```python
from build123d import *

# Parameters (mm, degrees)
F2_DEPTH = 12.7
F3_D     = 9.525


with BuildPart() as f2:
    # F1 (on Top) → F2 (new body)
    with BuildSketch(Plane.XY):
        with BuildLine():
            ThreePointArc((-122.0150568144, -68.2625), (-138.5539190608, -65.4948436404), (-153.2906597609, -57.4934462832))
            Line((-153.2906597609, -57.4934462832), (-236.4102435549, 7.4466898162))
            ThreePointArc((-236.4102435549, 7.4466898162), (-234.1628787728, 4.6714254371), (-233.3595565153, 1.1918544595))
            ThreePointArc((-233.3595565153, 1.1918544595), (-237.8174855377, -5.942323283), (-246.1838694757, -5.0629808973))
            Line((-246.1838694757, -5.0629808973), (-163.0642856817, -70.0031169967))
            ThreePointArc((-163.0642856817, -70.0031169967), (-143.7223135128, -80.5049510281), (-122.0150568144, -84.1375))
            Line((-122.0150568144, -84.1375), (-33.3375, -84.1375))
            ThreePointArc((-33.3375, -84.1375), (-4.1516676065, -72.0483323935), (7.9375, -42.8625))
            Line((7.9375, -42.8625), (7.9375, 0))
            ThreePointArc((7.9375, 0), (0, -7.9375), (-7.9375, 0))
            Line((-7.9375, 0), (-7.9375, -42.8625))
            ThreePointArc((-7.9375, -42.8625), (-15.3769877579, -60.8230122421), (-33.3375, -68.2625))
            Line((-33.3375, -68.2625), (-122.0150568144, -68.2625))
        make_face()
        with BuildLine():
            ThreePointArc((-233.3595565153, 1.1918544595), (-234.1628787728, 4.6714254371), (-236.4102435549, 7.4466898162))
            ThreePointArc((-236.4102435549, 7.4466898162), (-247.5518918721, 6.0786674199), (-246.1838694757, -5.0629808973))
            ThreePointArc((-246.1838694757, -5.0629808973), (-237.8174855377, -5.942323283), (-233.3595565153, 1.1918544595))
        make_face()
        with BuildLine():
            ThreePointArc((7.9375, 0), (0, 7.9375), (-7.9375, 0))
            ThreePointArc((-7.9375, 0), (0, -7.9375), (7.9375, 0))
        make_face()
    extrude(amount=F2_DEPTH)

    # F3 (through all)
    with Locations(Plane(origin=(0, 0, 0), x_dir=(1, 0, 0), z_dir=(0, 0, -1))):
        with Locations((-241.2970565153, -1.1918544595), (0, 0)):
            Hole(F3_D / 2)


solid = f2.part
```
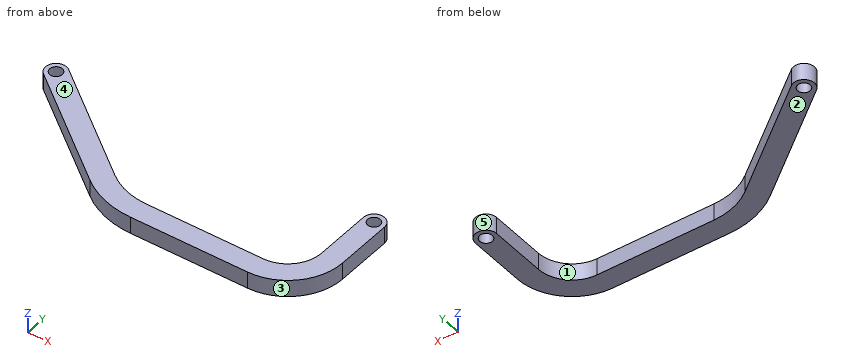
CAD build for the part. Positions are in the model's coordinates, mm. Face numbers are marked on the shaded views. A direction names the side the tool comes from. Round coordinates to 2 decimals unless told otherwise and drop trailing zeros. Order: outer loops, then holes, each group sorted by start corner. A loop starts at its lowest first (then second) coordinate and runs counter-clockwise, first axis right, second up.
Item 1: Saw through at D-D on x = -54. Write the cut outline in (y, z), then the cut area to 3 significant figures.
Item 2: Probe line 1 along Y through (x, z) = (-34.5, 6.25); line 2 along X through (y, z) = (-12.5, 1.5); line 3 along X through (y, z) = (-47.5, 1). List the from-to ranges inside material, lowest first.
Item 3: Saw through at A-A on x = 0. Write the cut outline in (y, z).
Item 4: Pin check, flat tip, straight feed: pin 1 (4 mm diameter, centred on x = -95.5, z = 5.5, fed in from +Y). Stop position of the tip, or through.
Item 5: Saw through at C-C on y = -17.5. Write the cut outline in (x, z), then the cut area to 3 significant figures.
Item 6: Saw through at B-B on z = 6. State how many separate pieces and enclosed holes the cut face has, then the cut area to 3 significant figures.
Item 7: Tool access for the marked faces 1 and 2: list every direction of +Z, -Z, +X, -X, +Y, -Y with a clear straight run to the whole face (end or side of a thin tool).
Item 8: Mould opens along X. For the marked faces 3, 4 and 5 say: pulls with the +X half, pulls with the -X half, needs draft (parallel to the pull), parting line crosses it, or undercut.
Reported:
1. outline: (-84.14, 0) - (-68.26, 0) - (-68.26, 12.7) - (-84.14, 12.7) - close
1. area: 202 mm2
2. line 1: y = -84.14 to -68.26
2. line 2: x = -236.66 to -210.88, -7.94 to 7.94
2. line 3: x = -191.87 to -166.08, -8.36 to 7.68
3. outline: (-67.2, 0) - (-4.76, 0) - (-4.76, 12.7) - (-67.2, 12.7) - close; (4.76, 0) - (7.94, 0) - (7.94, 12.7) - (4.76, 12.7) - close
4. pin 1: stops at y = -68.26
5. outline: (-230.27, 0) - (-204.48, 0) - (-204.48, 12.7) - (-230.27, 12.7) - close; (-7.94, 0) - (7.94, 0) - (7.94, 12.7) - (-7.94, 12.7) - close
5. area: 529 mm2
6. separate pieces: 1
6. enclosed holes: 2
6. area: 5,270 mm2
7. face 1: +Z, -Z, +Y
7. face 2: -Z, +X, -X, +Y, -Y
8. face 3: pulls with the +X half
8. face 4: needs draft
8. face 5: undercut
